CAD build for the part. Positions are in the model's coordinates, mm. A direction names the side the tool comes from. Coordinates: 2 decimals unless noted, no trailing zeros. Order: outer loops, then holes, each group sorted by start corner. A loop starts at its lowest first (then second) coordinate and runs counter-clockwise, first axis right, second up. Notation, with made-up numbers: (80, 68) - (87, 68) arc R15 cw to (87, 77) - close; hole circle Ø5 at (46, -5). An arc over 180 degrees is marked (long way). Use one line per item in the form item = value.
```python
from build123d import *

# Parameters (mm, degrees)
SKETCH1_W           = 15.85
SKETCH1_H           = 15.85
BOSS_EXTRUDE1_DEPTH = 3.18
SKETCH2_R           = 2.35
BOSS_EXTRUDE2_DEPTH = 1.96
SHELL1_T            = -1.38
SKETCH3_R           = 3.1
SKETCH3_R_2         = 2.82
BOSS_EXTRUDE3_DEPTH = 1.48


with BuildPart() as part:
    # Sketch1 → Boss-Extrude1 (new body)
    with BuildSketch(Plane(origin=(0, 0, 0), x_dir=(1, 0, 0), z_dir=(0, 1, 0))):
        Rectangle(SKETCH1_W, SKETCH1_H)
    extrude(amount=-BOSS_EXTRUDE1_DEPTH)

    # Sketch2 → Boss-Extrude2 (add)
    with BuildSketch(Plane(origin=(0, 0, 0), x_dir=(1, 0, 0), z_dir=(0, 1, 0))):
        with Locations(Location((-4.065, -3.9625, 0), (0, 0, 270))):
            Circle(SKETCH2_R)
        with Locations(Location((4.065166585, -3.9625, 0), (0, 0, 270))):
            Circle(SKETCH2_R)
    extrude(amount=BOSS_EXTRUDE2_DEPTH)

    # Shell1
    shell1_openings = [part.faces().sort_by_distance(p)[0] for p in [
        (0, -3.18, 0),
    ]]
    offset(amount=SHELL1_T, openings=shell1_openings, kind=Kind.INTERSECTION)

    # Sketch3 → Boss-Extrude3 (add)
    with BuildSketch(Plane.XZ.offset(1.38)):
        with Locations(Location((0, 0, 0), (0, 0, 90))):
            Circle(SKETCH3_R)
        with Locations(Location((0, 0, 0), (0, 0, 270))):
            Circle(SKETCH3_R_2, mode=Mode.SUBTRACT)
    extrude(amount=BOSS_EXTRUDE3_DEPTH)


solid = part.part
```
Item 1: Drop flat-ended pins along their axis: pin 1 (8 mm diameter, centred on x = 3.5, z = -3, fed in from +Y); pin 2 (2 mm diameter, centred on x = -4.5, z = 3.5, fed in from -Y); pin 3 (1.6 mm diameter, centred on x = 4.07, z = 3.96, fed in from -Y). Give the stop position or say it passes through.
Derived:
pin_1 = 0
pin_2 = -1.38
pin_3 = 0.58
Item 2: Cut at B-B, the plane z = 0. Write the cut outline in (x, y) (3 decimals), plus the area to 3 significant figures.
Derived:
outline = (-7.925, -3.18) - (-6.545, -3.18) - (-6.545, -1.38) - (-3.1, -1.38) - (-3.1, -2.86) - (-2.82, -2.86) - (-2.82, -1.38) - (2.82, -1.38) - (2.82, -2.86) - (3.1, -2.86) - (3.1, -1.38) - (6.545, -1.38) - (6.545, -3.18) - (7.925, -3.18) - (7.925, 0) - (-7.925, 0) - close
area = 27.7 mm²
Item 3: Two-plate mould, pull along X, no slides. Class faces 1 (the face through (-4.022, -0.414, 2.993)), 2 (the face through (0, -2, -6.545)), 3 (the face through (0, -2, 7.925)), 4 (the face through (7.925, -2, 0)): +X half, -X half, draft (parallel to the pull), parting line (faces both ways), or undercut.
Derived:
face_1 = undercut
face_2 = undercut
face_3 = draft
face_4 = +X half
Item 4: Drill centre lines: line 1 (X direction, y = -2.95, z = -2.5) (3 decimals); line 2 (Z direction, x = -0.5, y = -2.1) (3 decimals). Where is each one in solid material? Low to high. Write a range as [from, to].
Derived:
line_1 = [-7.925, -6.545], [6.545, 7.925]
line_2 = [-7.925, -6.545], [-3.059, -2.775], [2.775, 3.059], [6.545, 7.925]
Item 5: Cut at D-D, the plane y = -0.35. Write the cut outline in (x, z) (1 decimal), plus the area to 3 significant figures.
Derived:
outline = (-7.9, -7.9) - (7.9, -7.9) - (7.9, 7.9) - (-7.9, 7.9) - close; hole circle Ø1.9 at (-4.1, 4); hole circle Ø1.9 at (4.1, 4)
area = 245 mm²
Item 6: 3-axis set-ups, long thin cutter, end or side, ignore diameter. For faces 5 (the face through (0, -2, -7.925)), 6 (the face through (0, -1.38, 0)), 7 (the face through (-3.962, 0.966, 1.615)): which of +Z, -Z, +X, -X, +Y, -Y reach the whole face in a straight line?
Derived:
face_5 = -Z, +X, -X, +Y, -Y
face_6 = -Y
face_7 = +Y
Item 7: Cut at C-C, the plane x = -3.75. Write the cut outline in (y, z) (3 decimals).
Derived:
outline = (-3.18, -7.925) - (0, -7.925) - (0, 1.634) - (1.96, 1.634) - (1.96, 6.291) - (0, 6.291) - (0, 7.925) - (-3.18, 7.925) - (-3.18, 6.545) - (-1.38, 6.545) - (-1.38, 4.88) - (0.58, 4.88) - (0.58, 3.045) - (-1.38, 3.045) - (-1.38, -6.545) - (-3.18, -6.545) - close
Item 8: Cut at A-A, the plane y = -1.65. Write the cut outline in (x, z) (3 decimals).
Derived:
outline = (-7.925, -7.925) - (7.925, -7.925) - (7.925, 7.925) - (-7.925, 7.925) - close; circle Ø6.2 at (0, 0); hole (-6.545, -6.545) - (6.545, -6.545) - (6.545, 6.545) - (-6.545, 6.545) - close; hole circle Ø5.64 at (0, 0)
